Source: CAD feature listing. Evaluate the final solid. Frame: model axes, mm. A direction names the side the tool comes from. Coordinates: 2 decimals unless noted, no trailing zeros. Loops run counter-clockwise (first coordinate to the right, second up) from the corner with the lowest first, then second, coordinate; pieces in that order, holes last. Notation, with made-up numbers: (1.5, 73) -> (25.5, 73) arc R24 ccw to (25.5, 101) -> close; hole circle Ø1 at (30.5, -35). An arc over 180 degrees is marked (long way). Answer as CSV lines item,"result".
from build123d import *

# Parameters (mm, degrees)
F0_R     = 3.81
F0_R_2   = 2.5
F0_R_3   = 3.3
F0_R_4   = 1.72466
F0_R_5   = 3.175
F0_R_6   = 50.8
F1_DEPTH = 1.5875
F2_R     = 6.34999


# Not quite as in the source:
# - a fillet or chamfer is up to 0.001 mm smaller than in the source, because OpenCascade refuses the exact size


with BuildPart() as f1:
    # F0 (on Front) → F1 (new body)
    with BuildSketch(Plane.XZ):
        with BuildLine():
            Line((-6.35, 207.9625), (-19.05, 207.9625))
            Line((-19.05, 207.9625), (-19.05, 191.187323006))
            Line((-19.05, 191.187323006), (13.4939129862, 172.0272456399))
            ThreePointArc((13.4939129862, 172.0272456399), (51.0340994838, 106.3625), (13.4939129862, 40.6977543601))
            Line((13.4939129862, 40.6977543601), (-19.05, 21.537676994))
            Line((-19.05, 21.537676994), (-19.05, 4.7625))
            Line((-19.05, 4.7625), (-6.35, 4.7625))
            Line((-6.35, 4.7625), (-6.35, -7.9375))
            Line((-6.35, -7.9375), (31.0143905041, -7.9375))
            Line((31.0143905041, -7.9375), (83.7986667883, 23.1389970933))
            ThreePointArc((83.7986667883, 23.1389970933), (96.215342788, 28.3751822993), (109.5718757899, 30.1625))
            Line((109.5718757899, 30.1625), (240.6114472101, 30.1625))
            ThreePointArc((240.6114472101, 30.1625), (253.967980212, 28.3751822993), (266.3846562117, 23.1389970933))
            Line((266.3846562117, 23.1389970933), (319.1689324959, -7.9375))
            Line((319.1689324959, -7.9375), (356.533323, -7.9375))
            Line((356.533323, -7.9375), (356.533323, 4.7625))
            Line((356.533323, 4.7625), (369.233323, 4.7625))
            Line((369.233323, 4.7625), (369.233323, 21.537676994))
            Line((369.233323, 21.537676994), (336.6894100138, 40.6977543601))
            ThreePointArc((336.6894100138, 40.6977543601), (299.1492235162, 106.3625), (336.6894100138, 172.0272456399))
            Line((336.6894100138, 172.0272456399), (369.233323, 191.187323006))
            Line((369.233323, 191.187323006), (369.233323, 207.9625))
            Line((369.233323, 207.9625), (356.533323, 207.9625))
            Line((356.533323, 207.9625), (356.533323, 220.6625))
            Line((356.533323, 220.6625), (319.1689324959, 220.6625))
            Line((319.1689324959, 220.6625), (266.3846562117, 189.5860029067))
            ThreePointArc((266.3846562117, 189.5860029067), (253.967980212, 184.3498177007), (240.6114472101, 182.5625))
            Line((240.6114472101, 182.5625), (109.5718757899, 182.5625))
            ThreePointArc((109.5718757899, 182.5625), (96.215342788, 184.3498177007), (83.7986667883, 189.5860029067))
            Line((83.7986667883, 189.5860029067), (31.0143905041, 220.6625))
            Line((31.0143905041, 220.6625), (-6.35, 220.6625))
            Line((-6.35, 220.6625), (-6.35, 207.9625))
        make_face()
        Circle(F0_R, mode=Mode.SUBTRACT)
        with Locations((-12.7, 12.7)):
            Circle(F0_R, mode=Mode.SUBTRACT)
        with Locations((0, 12.7)):
            Circle(F0_R, mode=Mode.SUBTRACT)
        with Locations((130.0916615, 46.3625)):
            Circle(F0_R_2, mode=Mode.SUBTRACT)
        with Locations((115.0916615, 61.3625)):
            Circle(F0_R_2, mode=Mode.SUBTRACT)
        with Locations((130.0916615, 61.3625)):
            Circle(F0_R_3, mode=Mode.SUBTRACT)
        with Locations((220.0916615, 46.3625)):
            Circle(F0_R_2, mode=Mode.SUBTRACT)
        with Locations((257.7919761398, 44.3280112686)):
            Circle(F0_R_4, mode=Mode.SUBTRACT)
        with Locations((319.6223383993, 7.9256731426)):
            Circle(F0_R_4, mode=Mode.SUBTRACT)
        with Locations((350.183323, 0)):
            Circle(F0_R, mode=Mode.SUBTRACT)
        with Locations((350.183323, 12.7)):
            Circle(F0_R, mode=Mode.SUBTRACT)
        with Locations((362.883323, 12.7)):
            Circle(F0_R, mode=Mode.SUBTRACT)
        Polygon((314.5229509507, 3.6403531184), (256.5190923021, 37.7898550455), (274.5603386032, 68.4334030108), (332.5641972518, 34.2839010837), align=None, mode=Mode.SUBTRACT)
        with Locations((331.2913134141, 27.7457448606)):
            Circle(F0_R_4, mode=Mode.SUBTRACT)
        with Locations((220.0916615, 61.3625)):
            Circle(F0_R_3, mode=Mode.SUBTRACT)
        with Locations((235.0916615, 61.3625)):
            Circle(F0_R_2, mode=Mode.SUBTRACT)
        with Locations((269.4609511546, 64.1480829866)):
            Circle(F0_R_4, mode=Mode.SUBTRACT)
        with Locations((115.0916615, 151.3625)):
            Circle(F0_R_2, mode=Mode.SUBTRACT)
        with Locations((130.0916615, 151.3625)):
            Circle(F0_R_3, mode=Mode.SUBTRACT)
        with Locations((-12.7, 200.025)):
            Circle(F0_R_5, mode=Mode.SUBTRACT)
        with Locations((0, 200.025)):
            Circle(F0_R_5, mode=Mode.SUBTRACT)
        with Locations((0, 212.725)):
            Circle(F0_R_5, mode=Mode.SUBTRACT)
        with Locations((130.0916615, 166.3625)):
            Circle(F0_R_2, mode=Mode.SUBTRACT)
        with Locations((175.0916615, 106.3625)):
            Circle(F0_R_6, mode=Mode.SUBTRACT)
        with Locations((220.0916615, 151.3625)):
            Circle(F0_R_3, mode=Mode.SUBTRACT)
        with Locations((235.0916615, 151.3625)):
            Circle(F0_R_2, mode=Mode.SUBTRACT)
        with Locations((220.0916615, 166.3625)):
            Circle(F0_R_2, mode=Mode.SUBTRACT)
        with Locations((350.183323, 200.025)):
            Circle(F0_R_5, mode=Mode.SUBTRACT)
        with Locations((362.883323, 200.025)):
            Circle(F0_R_5, mode=Mode.SUBTRACT)
        with Locations((350.183323, 212.725)):
            Circle(F0_R_5, mode=Mode.SUBTRACT)
    extrude(amount=F1_DEPTH)

    # F2 (radius 6.35 in the source; OpenCascade refuses exactly that, so slightly less here)
    f2_edges = [f1.edges().sort_by_distance(p)[0] for p in [
        (-6.35, -0.79375, 207.9625),
        (-6.35, -0.79375, 220.6625),
        (-19.05, -0.79375, 207.9625),
        (356.533323, -0.79375, 207.9625),
        (356.533323, -0.79375, 220.6625),
        (369.233323, -0.79375, 207.9625),
        (356.533323, -0.79375, 4.7625),
        (369.233323, -0.79375, 4.7625),
        (356.533323, -0.79375, -7.9375),
        (-6.35, -0.79375, 4.7625),
        (-19.05, -0.79375, 4.7625),
        (-6.35, -0.79375, -7.9375),
    ]]
    fillet(f2_edges, radius=F2_R)


solid = f1.part
(1) Cut plane D-D (x = 91.5). Return the cut outline in (y, z).
Computed values:
outline,"(-1.59, 26.84) -> (0, 26.84) -> (0, 185.89) -> (-1.59, 185.89) -> close"
(2) Access query for faces 5 (the flat face through (265.413, -0.783, 52.897)), 6 (the cylindrical face through (96.4, -0.8, 184.3)), 7 (the cylindrical face through (96.033, -0.783, 28.325)). Directions: +Z, -Z, +X, -X, +Y, -Y. A direction counts if a zero-diameter tool reaches every point of the face in a straight line with its end or side. Return the directions, or none.
Computed values:
face 5,"+Y, -Y"
face 6,"+Z, +Y, -Y"
face 7,"-Z, +Y, -Y"
(3) Cut plane A-A (z = 131). Return the cut outline in (x, y), then the cut area to 3 significant figures.
Computed values:
outline,"(46.94, -1.59) -> (130.67, -1.59) -> (130.67, 0) -> (46.94, 0) -> close; (219.52, -1.59) -> (303.24, -1.59) -> (303.24, 0) -> (219.52, 0) -> close"
area,"266 mm^2"
(4) Draft query along X for faces 1 (the flat face through (353.189, -0.783, 30.984)), 2 (the flat face through (-2.55, -0.78, 31.25)), 3 (the cylindrical face through (253.785, -0.783, 28.425)), 4 (the flat face through (129, -1.588, 83)). Return one class per face: released by +X, released by -X, zero draft, split by the parting line, or undercut.
Computed values:
face 1,"released by +X"
face 2,"released by -X"
face 3,"undercut"
face 4,"zero draft"
(5) Cut plane B-B (z = 79.5). Return the cut outline in (x, y) (1 decimal), then the cut area to 3 significant figures.
Computed values:
outline,"(46.1, -1.6) -> (132, -1.6) -> (132, 0) -> (46.1, 0) -> close; (218.2, -1.6) -> (304, -1.6) -> (304, 0) -> (218.2, 0) -> close"
area,"273 mm^2"
(6) Cut plane C-C (y = -0.3). State how many separate pieces and enclosed holes the cut face has, then the cut area to 3 significant figures.
Computed values:
separate pieces,"1"
enclosed holes,"30"
area,"43,000 mm^2"
(7) Material intervals for L1, parallel to Z at x = 221.5, y = -0.45; L2, parallel to Z at x = 323.5, y = -0.85; L3, parallel to Z at x = 318.5, y = -0.2, sorted ascending. Write a range as [from, to].
Computed values:
L1,"[30.16, 44.3], [48.43, 58.38], [64.35, 85.7], [127.02, 148.38], [154.35, 164.3], [168.43, 182.56]"
L2,"[-7.94, 18.89], [39.62, 50.52], [162.2, 220.66]"
L3,"[-7.54, 6.62], [9.24, 10.4], [42.56, 55.62], [157.1, 220.27]"
